Model file for the job. Use its own axes, mm. A direction names the side the tool comes from. Give positions to 0.01 mm unless a question says otherwise; leave off trailing zeros. Order: outer loops, then holes, each group sorted by start corner. A loop starts at its lowest first (then second) coordinate and runs counter-clockwise, first axis right, second up. Notation, with made-up numbers: (87.5, 66.5) - (112.5, 66.5) arc R13 cw to (112.5, 70.5) - close; hole circle Ø6 at (42, 52). An arc over 180 degrees is marked (long way). Use CSV: the item, a comma, the result in double quotes. Start each with the question number.
(1) Tool access for faces 4 (the flat face through (16.053, 0, 0)), 5 (the flat face through (1, 0, 1.981)): list every direction of +Z, -Z, +X, -X, +Y, -Y with a clear straight run to the whole face (end or side of a thin tool).
(2) Band-saw the part on A-A, the plane x = 9.5. Give the cut face in (y, z) (3 decimals).
(3) Probe L1, parallel to X at y = -3.25, z = -2.75; L2, parallel to Y at x = 2, z = -1; L3, parallel to X at y = 1.5, z = 1. List the from-to ranges inside material, lowest first.
(4) Band-saw the part on B-B, the plane y = -4.25. Give the cut face in (x, z).
(5) Drop flat-ended pins along their axis: pin 1 Ø1.8 at (x, y) = (1.5, -0.5) entering from +Z; pin 2 Ø1 at (x, y) = (6.5, -1) entering from +Z; pin 3 Ø2.5 at (x, y) = (1, 0) entering from -Z. Give the stop position or say it passes through.
(6) Band-saw the part on C-C, the plane z = -4.5. Give the cut face in (x, y).
(7) Pull direction Y, two halves, no side cores. Call faces 1 (the flat face through (1, 0, -1.981)), 2 (the cylindrical face through (9.24, -0.69, -3.1)), 3 (the flat face through (3.353, -2.4, -2.4)): +Y half, -Y half, draft (parallel to the pull), parting line (faces both ways), or undercut.
from build123d import *

# Parameters (mm, degrees)
HEX_2_DEPTH = 2.2098


with BuildPart() as part:
    # BodySke → BaseBody (revolve)
    with BuildSketch(Plane.XY):
        with BuildLine():
            Line((16.0528, 0), (16.0528, 2.41935))
            Line((16.0528, 2.41935), (15.29715, 3.175))
            Line((15.29715, 3.175), (3.3528, 3.175))
            Line((3.3528, 3.175), (3.3528, 5.5499))
            Line((3.3528, 5.5499), (2.5654, 5.5499))
            ThreePointArc((2.5654, 5.5499), (1.073764503, 4.355582759), (0, 2.77495))
            Line((0, 2.77495), (0, 0))
            Line((0, 0), (16.0528, 0))
        make_face()
    revolve(axis=Axis((0, 0, 0), (1, 0, 0)))

    # Sketch2 → PreBroach (revolve, cut)
    with BuildSketch(Plane.XY):
        Polygon((0, 1.9812), (2.2098, 1.9812), (3.353646353, 0), (0, 0), align=None)
    revolve(axis=Axis((0, 0, 0), (1, 0, 0)), mode=Mode.SUBTRACT)

    # Sketch3 → Hex 2 (cut)
    with BuildSketch(Plane(origin=(0, 0, 0), x_dir=(0, 0, -1), z_dir=(1, 0, 0))):
        Polygon((-1.9812, -1.143846353), (-1.9812, 1.143846353), (0, 2.287692707), (1.9812, 1.143846353), (1.9812, -1.143846353), (0, -2.287692707), align=None)
    extrude(amount=HEX_2_DEPTH, mode=Mode.SUBTRACT)


solid = part.part
Answer block:
1,face 4,"+Z, -Z, +X, +Y, -Y"
1,face 5,"-X"
2,outline,"circle Ø6.35 at (0, 0)"
3,L1,"x = 0.98 to 3.35"
3,L2,"y = -5.08 to -1.71, 1.71 to 5.08"
3,L3,"x = 2.31 to 16.05"
4,outline,"(2.57, -3.57) - (3.35, -3.57) - (3.35, 3.57) - (2.57, 3.57) arc R4.81 ccw to start"
5,pin 1,"stops at z = 5.43"
5,pin 2,"stops at z = 3.14"
5,pin 3,"stops at z = -5.35"
6,outline,"(2.57, -3.25) - (3.35, -3.25) - (3.35, 3.25) - (2.57, 3.25) arc R4.57 ccw to start"
7,face 1,"undercut"
7,face 2,"parting line"
7,face 3,"draft"
